Geometry check sheet. Reference: the model listing, model coordinates, mm. Round coordinates to 2 decimals unless told otherwise and drop trailing zeros. Order: outer loops, then holes, each group sorted by start corner. A loop starts at its lowest first (then second) coordinate and runs counter-clockwise, first axis right, second up.
(1) Release check for a two-part mould opening along Z. For faces 1 (the face through (188.52, -2.96, -113.27)), 2 (the face through (180, 0, -77)) record: +Z half, -Z half, draft (parallel to the pull), parting line (faces both ways), or undercut.
(2) Material ranges on line 1 along Z through (x, y) = (174, -0.75); line 2 along Z through (x, y) = (147, -5.5); line 3 along Z through (x, y) = (178, -3.5), recorded low to high.
(3) Go/stop test with flat-tipped pins: pin 1 (3 mm diameter, centred on y = -3.5, z = -315, fed in from -X); pin 2 (4 mm diameter, centred on x = 156.5, z = 81.5, fed in from -Y); pin 3 (1.5 mm diameter, centred on x = 183.5, y = -2.5, fed in from +Z); pin 4 (3 mm diameter, centred on x = 149, y = -3.5, fed in from +Z). Record where each tip stops, or that it passes through.
(4) Sectioned sample at A-A (x = 168.5). Record the boundary of the cut face in (y, z), plus the area to 3 significant figures.
(5) Sectioned sample at B-B (y = -4). Give the number of separate pieces and of enclosed holes in the cut face, plus the area to 3 significant figures.
from build123d import *

# Parameters (mm, degrees)
F0_W     = 21.1715102196
F0_H     = 58.4797523916
F0_R     = 16.9272487263
F1_DEPTH = 6


with BuildPart() as f1:
    # F0 (on Front) → F1 (new body)
    with BuildSketch(Plane.XZ):
        with BuildLine():
            Line((203.8914743591, -81.3288328435), (203.8914743591, -80.4375457843))
            Line((203.8914743591, -80.4375457843), (174.4579714171, -80.4375457843))
            Line((174.4579714171, -80.4375457843), (174.4579714171, -85.4375457843))
            Line((174.4579714171, -85.4375457843), (144.4579714171, -85.4375457843))
            Line((144.4579714171, -85.4375457843), (144.4579714171, -303.4375457843))
            Line((144.4579714171, -303.4375457843), (154.4579714171, -303.4375457843))
            Line((154.4579714171, -303.4375457843), (154.4579714171, -323.4375457843))
            Line((154.4579714171, -323.4375457843), (178.2914743591, -323.4375457843))
            add(Edge.make_bspline(
                [(178.2914743591, -323.4375457843), (202.3683447271, -316.6747764881), (203.8304484738, -107.4468228501), (203.8914743591, -82.7989785763)],
                knots=[0, 0, 0, 0, 229.5065578532, 229.5065578532, 229.5065578532, 229.5065578532], degree=3))
            Line((203.8914743591, -82.7989785763), (203.8914743591, -81.3288328435))
        make_face()
        with Locations((166.0767396396, -262.2106793639)):
            Rectangle(F0_W, F0_H, mode=Mode.SUBTRACT)
        with Locations((172.373637557, -118.3564311424)):
            Circle(F0_R, mode=Mode.SUBTRACT)
        with BuildLine():
            add(Edge.make_bspline(
                [(203.8914743591, -78.0761129922), (203.895419842, -79.6696605209), (203.8935088751, -80.4916705159), (203.8914743591, -80.4375457843)],
                knots=[229.5065578531, 229.5065578531, 229.5065578531, 229.5065578531, 244.3447564406, 244.3447564406, 244.3447564406, 244.3447564406], degree=3))
            add(Edge.make_bspline(
                [(178.2914743591, 162.5624542157), (202.3683447271, 155.7996849196), (203.8304484738, -53.4282687183), (203.8914743591, -78.0761129922)],
                knots=[0, 0, 0, 0, 229.5065578531, 229.5065578531, 229.5065578531, 229.5065578531], degree=3))
            Line((178.2914743591, 162.5624542157), (154.4579714171, 162.5624542157))
            Line((154.4579714171, 162.5624542157), (154.4579714171, 142.5624542157))
            Line((154.4579714171, 142.5624542157), (144.4579714171, 142.5624542157))
            Line((144.4579714171, 142.5624542157), (144.4579714171, -75.4375457843))
            Line((144.4579714171, -75.4375457843), (174.4579714171, -75.4375457843))
            Line((174.4579714171, -75.4375457843), (174.4579714171, -80.4375457843))
            Line((174.4579714171, -80.4375457843), (203.8914743591, -80.4375457843))
        make_face()
        with Locations((172.373637557, -42.5186604261)):
            Circle(F0_R, mode=Mode.SUBTRACT)
        with Locations((166.0767396396, 101.3355877954)):
            Rectangle(F0_W, F0_H, mode=Mode.SUBTRACT)
        with BuildLine():
            Line((203.8914743591, -79.546258725), (203.8914743591, -78.0761129922))
            add(Edge.make_bspline(
                [(203.8914743591, -78.0761129922), (203.895419842, -79.6696605209), (203.8935088751, -80.4916705159), (203.8914743591, -80.4375457843)],
                knots=[229.5065578531, 229.5065578531, 229.5065578531, 229.5065578531, 244.3447564406, 244.3447564406, 244.3447564406, 244.3447564406], degree=3))
            Line((203.8914743591, -80.4375457843), (203.8914743591, -79.546258725))
        make_face(mode=Mode.SUBTRACT)
    extrude(amount=F1_DEPTH)


solid = f1.part
Answer below:
1. face 1: undercut
1. face 2: draft
2. line 1: z = -323.44 to -291.45, -232.97 to -135.21, -101.51 to -85.44, -75.44 to -59.37, -25.67 to 72.1, 130.58 to 162.56
2. line 2: z = -303.44 to -85.44, -75.44 to 142.56
2. line 3: z = -323.44 to -134.32, -102.39 to -58.48, -26.55 to 162.56
3. pin 1: stops at x = 154.46
3. pin 2: stops at y = -6
3. pin 3: stops at z = 158.72
3. pin 4: stops at z = 142.56
4. outline: (-6, -323.44) - (0, -323.44) - (0, -291.45) - (-6, -291.45) - close; (-6, -232.97) - (0, -232.97) - (0, -134.83) - (-6, -134.83) - close; (-6, -101.88) - (0, -101.88) - (0, -85.44) - (-6, -85.44) - close; (-6, -75.44) - (0, -75.44) - (0, -59) - (-6, -59) - close; (-6, -26.04) - (0, -26.04) - (0, 72.1) - (-6, 72.1) - close; (-6, 130.58) - (0, 130.58) - (0, 162.56) - (-6, 162.56) - close
4. area: 1,760 mm2
5. separate pieces: 1
5. enclosed holes: 4
5. area: 21,300 mm2
